Input: part model. Units: mm. Frame: model coordinates. Face numbers are marked on the shaded views. Round coordinates to 2 decimals unless told otherwise and drop trailing zeros. Order: outer loops, then holes, each group sorted by start corner. A loop starts at its lowest first (then second) coordinate and runs counter-clockwise, first axis right, second up. Notation, with made-up numbers: (65, 33) -> (74, 33) arc R37 cw to (74, 69) -> close; hole circle Ø9 at (-16, -33.75). An arc over 180 degrees is marked (long way). Answer as CSV lines item,"result". Start each with the question number.
1) Section query A-A, the plane y = 40. Output: boundary loops of the cut face in (x, z), and give its area (3 significant figures).
2) Line query: L1, parallel to X at y = 49, z = 1.75; L2, parallel to X at y = 20.5, z = 5.5; L3, parallel to Y at x = 67.5, z = 6.75. Output: solid intervals per line, ascending.
3) Mould query, pull axis X, two halves, no side actions, for the marked faces 1, 2 and 3. Classes: +X half, -X half, draft (parallel to the pull), parting line (faces both ways), or undercut.
4) First-contact query: P1, Ø6, axis at y = 15.5, z = 5, coming from the -X side. Flat tip, straight axial feed; report the tip coordinate or a pass-through.
5) Section query B-B, the plane z = 6.75. Output: boundary loops of the cut face in (x, y), and give its area (3 significant figures).
6) Section query D-D, the plane x = 26. State how many separate pieces and enclosed holes the cut face has, and give its area (3 significant figures).
7) Section query C-C, the plane x = 45. Output: boundary loops of the cut face in (y, z).
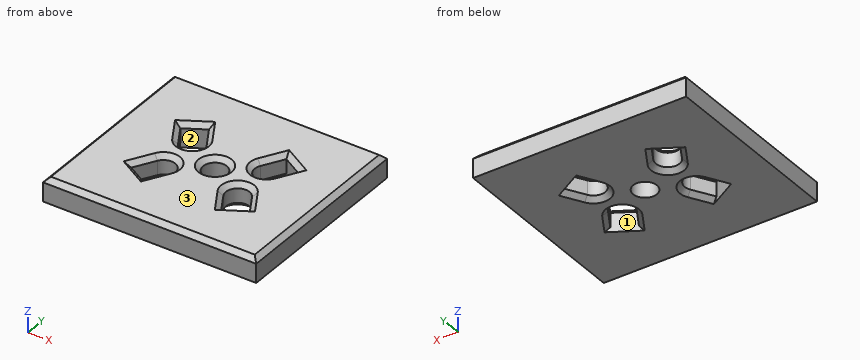
```python
from build123d import *

# Parameters (mm, degrees)
SKETCH_W      = 90
SKETCH_H      = 80
SKETCH_R      = 5
EXTRUDE_DEPTH = 10
CHAMFER_SIZE  = 2


with BuildPart() as part:
    # Sketch → Extrude (new body)
    with BuildSketch(Plane.XY):
        with Locations((45, 40)):
            Rectangle(SKETCH_W, SKETCH_H)
        with Locations((45, 40)):
            Circle(SKETCH_R, mode=Mode.SUBTRACT)
        with BuildLine():
            Line((28.660254, 60), (33.660254, 51.339746))
            ThreePointArc((25, 46.339746), (31.830127, 44.509619), (33.660254, 51.339746))
            Line((25, 46.339746), (20, 55))
            Line((20, 55), (28.660254, 60))
        make_face(mode=Mode.SUBTRACT)
        with BuildLine():
            Line((56.339746, 51.339746), (61.339746, 60))
            Line((61.339746, 60), (70, 55))
            Line((70, 55), (65, 46.339746))
            ThreePointArc((56.339746, 51.339746), (58.169873, 44.509619), (65, 46.339746))
        make_face(mode=Mode.SUBTRACT)
        with BuildLine():
            Line((65, 33.660254), (70, 25))
            Line((70, 25), (61.339746, 20))
            Line((61.339746, 20), (56.339746, 28.660254))
            ThreePointArc((65, 33.660254), (58.169873, 35.490381), (56.339746, 28.660254))
        make_face(mode=Mode.SUBTRACT)
        with BuildLine():
            Line((20, 25), (25, 33.660254))
            ThreePointArc((33.660254, 28.660254), (31.830127, 35.490381), (25, 33.660254))
            Line((33.660254, 28.660254), (28.660254, 20))
            Line((28.660254, 20), (20, 25))
        make_face(mode=Mode.SUBTRACT)
    extrude(amount=EXTRUDE_DEPTH)

    # Chamfer
    chamfer_edges = [part.edges().sort_by_distance(p)[0] for p in [
        (45, 0, 10),
        (90, 40, 10),
        (45, 80, 10),
        (0, 40, 10),
        (31.160254, 24.330127, 0),
        (24.330127, 22.5, 10),
        (22.5, 29.330127, 10),
        (65, 33.660254, 5),
        (67.5, 29.330127, 0),
        (65.669873, 22.5, 10),
        (58.839746, 24.330127, 10),
        (56.339746, 51.339746, 5),
        (58.839746, 55.669873, 0),
        (65.669873, 57.5, 10),
        (67.5, 50.669873, 10),
        (25, 46.339746, 5),
        (22.5, 50.669873, 0),
        (24.330127, 57.5, 10),
        (31.160254, 55.669873, 10),
        (50, 40, 5),
        (40, 40, 10),
    ]]
    chamfer(chamfer_edges, length=CHAMFER_SIZE)


solid = part.part
```
Findings:
1,outline,"(0, 0) -> (40, 0) -> (40, 8) -> (38, 10) -> (2, 10) -> (0, 8) -> close; (50, 0) -> (90, 0) -> (90, 8) -> (88, 10) -> (52, 10) -> (50, 8) -> close"
1,area,"792 mm^2"
2,L1,"x = 0 to 23.18, 34.58 to 55.42, 66.82 to 90"
2,L2,"x = 0 to 27.79, 28.95 to 61.05, 62.21 to 90"
2,L3,"y = 0 to 23.56, 29.33 to 50.67, 56.44 to 80"
3,face 1,"undercut"
3,face 2,"undercut"
3,face 3,"draft"
4,P1,"stops at x = 0"
5,outline,"(0, 0) -> (90, 0) -> (90, 80) -> (0, 80) -> close; hole (20, 25) -> (28.66, 20) -> (33.66, 28.66) arc R5 ccw to (25, 33.66) -> close; hole (20, 55) -> (25, 46.34) arc R5 ccw to (33.66, 51.34) -> (28.66, 60) -> close; hole circle Ø10 at (45, 40); hole (56.34, 28.66) -> (61.34, 20) -> (70, 25) -> (65, 33.66) arc R5 ccw to start; hole (56.34, 51.34) arc R5 ccw to (65, 46.34) -> (70, 55) -> (61.34, 60) -> close"
5,area,"6,560 mm^2"
6,separate pieces,"3"
6,enclosed holes,"0"
6,area,"514 mm^2"
7,outline,"(0, 0) -> (35, 0) -> (35, 8) -> (33, 10) -> (2, 10) -> (0, 8) -> close; (45, 0) -> (80, 0) -> (80, 8) -> (78, 10) -> (47, 10) -> (45, 8) -> close"
